Source: three-view drawing plus pictorial views. Frame: mm from the lowest corner of the part. Coordinates: 2 decimals unless noted, no trailing zeros. Write each loop counter-clockwise with the first axis right and the second up, starting at its lowest first coordinate (ties: lowest second). Pieces come first, ordered by that corner, then holes. Notation, with made-up numbers: (-21, 52.5) - (12, 52.5) arc R12 ccw to (12, 68.5) - close; hole circle Ø10 at (4.5, 42). An arc over 180 degrees is marked (long way). Put each result on its own line as item: value.
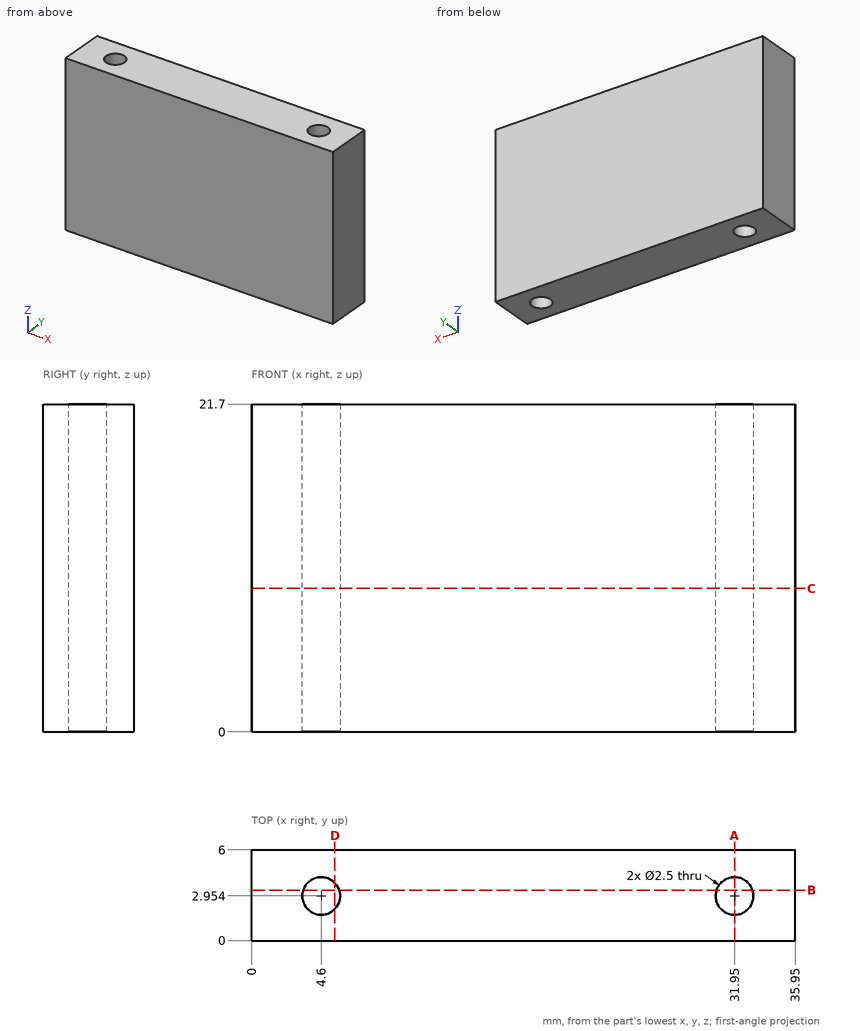
1. Section query A-A (x = 31.95). Return loops of the section in (y, z).
Answer below:
outline: (0, 0) - (1.7, 0) - (1.7, 21.7) - (0, 21.7) - close; (4.2, 0) - (6, 0) - (6, 21.7) - (4.2, 21.7) - close
2. Section query D-D (x = 5.5). Return loops of the section in (y, z).
Answer below:
outline: (0, 0) - (2.09, 0) - (2.09, 21.7) - (0, 21.7) - close; (3.82, 0) - (6, 0) - (6, 21.7) - (3.82, 21.7) - close
3. Ray query, probe 1 along Y at (x, z) = (31.95, 5.5); probe 2 along X at (y, z) = (3.55, 20); probe 3 along X at (y, z) = (3.3, 1.25). Return the intervals inside material, ascending. Write a range as from..to.
Answer below:
probe 1: y = 0..1.7, 4.2..6
probe 2: x = 0..3.5, 5.7..30.85, 33.05..35.95
probe 3: x = 0..3.4, 5.8..30.75, 33.15..35.95
4. Pin query (flat end, axial travel): pin 1 Ø2 at (x, y) = (5, 2) entering from -Z; pin 2 Ø2 at (x, y) = (31.95, 2.95) entering from -Z. Return the tip coordinate at first contact, or that it passes through.
Answer below:
pin 1: stops at z = 0
pin 2: passes through
5. Section query C-C (z = 9.5). Return loops of the section in (x, y), then the cut area to 3 significant figures.
Answer below:
outline: (0, 0) - (35.95, 0) - (35.95, 6) - (0, 6) - close; hole circle Ø2.5 at (4.6, 2.95); hole circle Ø2.5 at (31.95, 2.95)
area: 206 mm²
6. Section query B-B (y = 3.35). Return loops of the section in (x, z), then the cut area to 3 significant figures.
Answer below:
outline: (0, 0) - (3.41, 0) - (3.41, 21.7) - (0, 21.7) - close; (5.79, 0) - (30.76, 0) - (30.76, 21.7) - (5.79, 21.7) - close; (33.14, 0) - (35.95, 0) - (35.95, 21.7) - (33.14, 21.7) - close
area: 677 mm²
